Work out the finished part from the listing and answer in its coordinate system (mm). Give positions to 0.01 mm unless a question says otherwise; leave off trailing zeros. Write each loop counter-clockwise with the first axis right and the second up, starting at its lowest first coordinate (ties: lowest second). Pieces come first, ordered by that corner, then holes. Notation, with made-up numbers: (78, 87) -> (125, 87) arc R32 ccw to (125, 126) -> close; hole circle Ø6 at (-28.75, 75). An arc over 180 degrees is marked (long way). Write item = value, one per line. Start each with the question number.
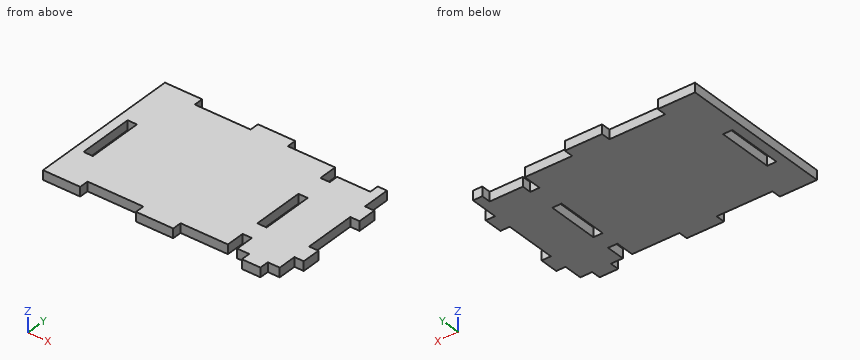
from build123d import *

# Parameters (mm, degrees)
ESQUISSE1_W             = 128.311788567
ESQUISSE1_H             = 73
BOSS_EXTRU_1_DEPTH      = 5
ESQUISSE3_W             = 5
ESQUISSE3_H             = 10
ESQUISSE3_H_2           = 28
ESQUISSE3_H_3           = 15
ESQUISSE3_H_4           = 30
ENL_V_MAT_EXTRU_1_DEPTH = 5
ESQUISSE4_W             = 17.86
ESQUISSE4_H             = 5
ENL_V_MAT_EXTRU_2_DEPTH = 5
ESQUISSE5_W             = 20
ESQUISSE5_H             = 5
ESQUISSE5_W_2           = 10
BOSS_EXTRU_2_DEPTH      = 5


with BuildPart() as part:
    # Esquisse1 → Boss.-Extru.1 (new body)
    with BuildSketch(Plane.XY):
        with Locations((-207.112987496, -6.063856407)):
            Rectangle(ESQUISSE1_W, ESQUISSE1_H)
    extrude(amount=BOSS_EXTRU_1_DEPTH)

    # Esquisse3 → Enlèv. mat.-Extru.1 (cut)
    with BuildSketch(Plane(origin=(0, 0, 0), x_dir=(-1, 0, 0), z_dir=(0, 0, -1))):
        with Locations((173.317093212, 25.436143593)):
            Rectangle(ESQUISSE3_W, ESQUISSE3_H)
        with Locations((173.317093212, -8.563856407)):
            Rectangle(ESQUISSE3_W, ESQUISSE3_H_2)
        with Locations((173.317093212, -37.563856407)):
            Rectangle(ESQUISSE3_W, ESQUISSE3_H)
        with Locations((145.457093212, 22.936143593)):
            Rectangle(ESQUISSE3_W, ESQUISSE3_H_3)
        with Locations((145.457093212, -8.563856407)):
            Rectangle(ESQUISSE3_W, ESQUISSE3_H_2)
        with Locations((145.457093212, -37.563856407)):
            Rectangle(ESQUISSE3_W, ESQUISSE3_H)
        with Locations((263.768881779, -11.288856407)):
            Rectangle(ESQUISSE3_W, ESQUISSE3_H_4)
    extrude(amount=-ENL_V_MAT_EXTRU_1_DEPTH, mode=Mode.SUBTRACT)

    # Esquisse4 → Enlèv. mat.-Extru.2 (cut)
    with BuildSketch(Plane.XY.offset(5)):
        with Locations((-161.887093212, 27.936143593)):
            Rectangle(ESQUISSE4_W, ESQUISSE4_H)
    extrude(amount=-ENL_V_MAT_EXTRU_2_DEPTH, mode=Mode.SUBTRACT)

    # Esquisse5 → Boss.-Extru.2 (add)
    with BuildSketch(Plane(origin=(0, 0, 0), x_dir=(-1, 0, 0), z_dir=(0, 0, -1))):
        with Locations((211.268881779, 32.936143593)):
            Rectangle(ESQUISSE5_W, ESQUISSE5_H)
        with Locations((261.268881779, 32.936143593)):
            Rectangle(ESQUISSE5_W, ESQUISSE5_H)
        with Locations((261.268881779, -45.063856407)):
            Rectangle(ESQUISSE5_W, ESQUISSE5_H)
        with Locations((211.268881779, -45.063856407)):
            Rectangle(ESQUISSE5_W, ESQUISSE5_H)
        with Locations((159.387093212, -45.063856407)):
            Rectangle(ESQUISSE5_W_2, ESQUISSE5_H)
    extrude(amount=-BOSS_EXTRU_2_DEPTH)


solid = part.part
(1) Find the intervals of material crossed by line 1 along X through (y, z) = (-7.5, 4.5); line 2 along X through (y, z) = (23.5, 4); line 3 along Y through (x, z) = (-174.5, 4.55), in increasing order.
(2) A cutting plane is placed at D-D, the plane x = -192.5. Write down the section's boundary in (y, z), then the cut area to 3 significant figures.
(3) A cutting plane is placed at C-C, the plane z = 2.4. State how many separate pieces and enclosed holes the cut face has, then the cut area to 3 significant figures.
(4) A cutting plane is placed at B-B, the plane y = -34. Write down the section's boundary in (x, z).
(5) Each of these flat-tipped pins is pushed along its axis until it touches: pin 1 (1.5 mm diameter, centred on x = -164.5, z = 3.5, fed in from +Y); pin 2 (1.5 mm diameter, centred on y = -39.5, z = 2, fed in from +X); pin 3 (1.5 mm diameter, centred on x = -145, z = 3.5, fed in from -Y). Where does it stop, or does it pass through?
(6) A cutting plane is placed at A-A, the plane y = -16.5. Write down the section's boundary in (x, z), then the cut area to 3 significant figures.
Results list:
q1.line_1 = -271.27 to -266.27, -261.27 to -175.82, -170.82 to -147.96
q1.line_2 = -271.27 to -175.82, -170.82 to -147.96
q1.line_3 = -32.56 to -22.56, 5.44 to 20.44
q2.outline = (-42.56, 0) -> (30.44, 0) -> (30.44, 5) -> (-42.56, 5) -> close
q2.area = 365 mm²
q3.separate_pieces = 1
q3.enclosed_holes = 2
q3.area = 9,070 mm²
q4.outline = (-271.27, 0) -> (-175.82, 0) -> (-175.82, 5) -> (-271.27, 5) -> close; (-170.82, 0) -> (-147.96, 0) -> (-147.96, 5) -> (-170.82, 5) -> close
q5.pin_1 = 25.44
q5.pin_2 = -147.96
q5.pin_3 = -32.56
q6.outline = (-271.27, 0) -> (-266.27, 0) -> (-266.27, 5) -> (-271.27, 5) -> close; (-261.27, 0) -> (-175.82, 0) -> (-175.82, 5) -> (-261.27, 5) -> close; (-170.82, 0) -> (-147.96, 0) -> (-147.96, 5) -> (-170.82, 5) -> close
q6.area = 567 mm²
